Design review of the part built by this model. Coordinates are the model's own, in mm. A direction names the side the tool comes from. Give positions to 0.01 mm unless a question says otherwise; leave off trailing zeros. Write each loop counter-clockwise with the first axis right and the second up, starting at its lowest first coordinate (ties: lowest second). Pieces come first, ordered by that corner, then holes. Notation, with made-up numbers: (-3.5, 87.5) -> (10.5, 87.5) arc R17 ccw to (10.5, 108.5) -> close; hole circle Ø11 at (0.5, 66.25). An arc over 180 degrees is marked (long way). Answer as a JSON object with one key per item and string values.
```python
from build123d import *

# Parameters (mm, degrees)
CROQUIS1_W              = 131.8
CROQUIS1_H              = 161.8
SALIENTE_EXTRUIR1_DEPTH = 9
CROQUIS2_W              = 124.8
CROQUIS2_H              = 154.8
SALIENTE_EXTRUIR2_DEPTH = 5
CROQUIS4_W              = 120.8
CROQUIS4_H              = 150.8
CORTAR_EXTRUIR1_DEPTH   = 10
REDONDEO1_R             = 4
REDONDEO2_R             = 2
REDONDEO3_R             = 4
REDONDEO4_R             = 4
REDONDEO5_R             = 2
REDONDEO6_R             = 4
REDONDEO7_R             = 2
REDONDEO8_R             = 6
CROQUIS9_W              = 124.8
CROQUIS9_H              = 2.5
CORTAR_EXTRUIR3_DEPTH   = 5
CROQUIS11_R             = 1.5
CORTAR_EXTRUIR6_DEPTH   = 9


with BuildPart() as part:
    # Croquis1 → Saliente-Extruir1 (new body)
    with BuildSketch(Plane.XY):
        with Locations((65.9, -80.9)):
            Rectangle(CROQUIS1_W, CROQUIS1_H)
    extrude(amount=SALIENTE_EXTRUIR1_DEPTH)

    # Croquis2 → Saliente-Extruir2 (add)
    with BuildSketch(Plane(origin=(0, 0, 0), x_dir=(-1, 0, 0), z_dir=(0, 0, -1))):
        with Locations((-65.9, -80.9)):
            Rectangle(CROQUIS2_W, CROQUIS2_H)
    extrude(amount=SALIENTE_EXTRUIR2_DEPTH)

    # Croquis4 → Cortar-Extruir1 (cut)
    with BuildSketch(Plane(origin=(0, 0, -5), x_dir=(-1, 0, 0), z_dir=(0, 0, -1))):
        with Locations((-65.9, -80.9)):
            Rectangle(CROQUIS4_W, CROQUIS4_H)
    extrude(amount=-CORTAR_EXTRUIR1_DEPTH, mode=Mode.SUBTRACT)

    # Redondeo1
    redondeo1_edges = [part.edges().sort_by_distance(p)[0] for p in [
        (128.3, -3.5, -2.5),
    ]]
    fillet(redondeo1_edges, radius=REDONDEO1_R)

    # Redondeo2
    redondeo2_edges = [part.edges().sort_by_distance(p)[0] for p in [
        (5.5, -5.5, 0),
    ]]
    fillet(redondeo2_edges, radius=REDONDEO2_R)

    # Redondeo3
    redondeo3_edges = [part.edges().sort_by_distance(p)[0] for p in [
        (3.5, -3.5, -2.5),
    ]]
    fillet(redondeo3_edges, radius=REDONDEO3_R)

    # Redondeo4
    redondeo4_edges = [part.edges().sort_by_distance(p)[0] for p in [
        (3.5, -158.3, -2.5),
    ]]
    fillet(redondeo4_edges, radius=REDONDEO4_R)

    # Redondeo5
    redondeo5_edges = [part.edges().sort_by_distance(p)[0] for p in [
        (5.5, -156.3, 0),
    ]]
    fillet(redondeo5_edges, radius=REDONDEO5_R)

    # Redondeo6
    redondeo6_edges = [part.edges().sort_by_distance(p)[0] for p in [
        (128.3, -158.3, -2.5),
    ]]
    fillet(redondeo6_edges, radius=REDONDEO6_R)

    # Redondeo7
    redondeo7_edges = [part.edges().sort_by_distance(p)[0] for p in [
        (126.3, -156.3, 0),
        (126.3, -5.5, 0),
    ]]
    fillet(redondeo7_edges, radius=REDONDEO7_R)

    # Redondeo8
    redondeo8_edges = [part.edges().sort_by_distance(p)[0] for p in [
        (0, 0, 4.5),
        (131.8, 0, 4.5),
        (131.8, -161.8, 4.5),
        (0, -161.8, 4.5),
    ]]
    fillet(redondeo8_edges, radius=REDONDEO8_R)

    # Croquis9 → Cortar-Extruir3 (cut)
    with BuildSketch(Plane(origin=(0, 0, -5), x_dir=(-1, 0, 0), z_dir=(0, 0, -1))):
        with Locations((-65.9, -52.15)):
            Rectangle(CROQUIS9_W, CROQUIS9_H)
        with Locations((-65.9, -109.65)):
            Rectangle(CROQUIS9_W, CROQUIS9_H)
    extrude(amount=-CORTAR_EXTRUIR3_DEPTH, mode=Mode.SUBTRACT)

    # Croquis11 → Cortar-Extruir6 (cut)
    with BuildSketch(Plane(origin=(0, 0, 5), x_dir=(-1, 0, 0), z_dir=(0, 0, -1))):
        with Locations((-25, -78.4)):
            Circle(CROQUIS11_R)
        with Locations((-25, -83.4)):
            Circle(CROQUIS11_R)
        with Locations((-20.5, -83.4)):
            Circle(CROQUIS11_R)
        with Locations((-16, -83.4)):
            Circle(CROQUIS11_R)
        with Locations((-20.5, -78.4)):
            Circle(CROQUIS11_R)
        with Locations((-16, -78.4)):
            Circle(CROQUIS11_R)
    extrude(amount=-CORTAR_EXTRUIR6_DEPTH, mode=Mode.SUBTRACT)


solid = part.part
```
(1) For line 1 along Y through (x, z) = (16, 8.05); line 2 along X through (y, z) = (-78.4, 6.8); line 3 along X through (y, z) = (-134.5, 0.25), list the stretches that pass through material, from the lowest coordinate up.
Here are the results:
{"line 1": "y = -161.8 to -84.9, -81.9 to -79.9, -76.9 to 0", "line 2": "x = 0 to 14.5, 17.5 to 19, 22 to 23.5, 26.5 to 131.8", "line 3": "x = 0 to 5.5, 126.3 to 131.8"}
(2) Clearance check with flat-ended pins moving along their axes: pin 1 (0.6 mm diameter, centred on x = 4.5, z = -2, fed in from +Y); pin 2 (0.6 mm diameter, centred on x = 5, z = -3.5, fed in from -Y); pin 3 (1 mm diameter, centred on x = 63.5, z = -2.5, fed in from +Y). State where each tip first meets the part, or that it passes through.
Here are the results:
{"pin 1": "stops at y = -4.55", "pin 2": "stops at y = -157.64", "pin 3": "stops at y = -3.5"}
(3) We need section C-C, the plane x = 53. State the section outline as (y, z) points, then the cut area to 3 significant figures.
Here are the results:
{"outline": "(-161.8, 0) -> (-158.3, 0) -> (-158.3, -5) -> (-156.3, -5) -> (-156.3, 5) -> (-5.5, 5) -> (-5.5, -5) -> (-3.5, -5) -> (-3.5, 0) -> (0, 0) -> (0, 9) -> (-161.8, 9) -> close", "area": "722 mm²"}
(4) We need section A-A, the plane z = -2.5. Give the number of separate pieces and of enclosed holes in the cut face, then the cut area to 3 significant figures.
Here are the results:
{"separate pieces": "4", "enclosed holes": "0", "area": "1,070 mm²"}
(5) For faces 1 (the flat face through (67, -5.5, 0)), 2 (the flat face through (128.3, -30, -2)), 3 (the flat face through (3.5, -30, -2)), 4 (the flat face through (67, -158.3, -2)), list the 3-axis set-ups (+Z, -Z, +X, -X, +Y, -Y) from which the entire face can be reached by the end or side of a thin tool; tool diameter is ignored.
Here are the results:
{"face 1": "-Z", "face 2": "-Z, +X, +Y, -Y", "face 3": "-Z, -X, +Y, -Y", "face 4": "-Z, +X, -X, -Y"}
(6) The part is to be moulded in two halves that separate along X. For faces 5 (the cylindrical face through (4.703, -4.641, -2.535)), 6 (the flat face through (67, -156.3, 0)), 7 (the cylindrical face through (129.996, -160.089, 4.563)), 8 (the flat face through (65, -161.8, 4)), say which applies: +X half, -X half, draft (parallel to the pull), parting line (faces both ways), or undercut.
Here are the results:
{"face 5": "-X half", "face 6": "undercut", "face 7": "+X half", "face 8": "draft"}
(7) We need section B-B, the plane y = -148.5. State the section outline as (x, z) points, then the cut area to 3 significant figures.
Here are the results:
{"outline": "(0, 0) -> (3.5, 0) -> (3.5, -5) -> (5.5, -5) -> (5.5, 5) -> (126.3, 5) -> (126.3, -5) -> (128.3, -5) -> (128.3, 0) -> (131.8, 0) -> (131.8, 9) -> (0, 9) -> close", "area": "602 mm²"}
